For this review, use the dimensioned drawing (mm, ordinates from the lowest corner) and the shaded views. A direction names the side the tool comes from. Coordinates: 2 decimals unless noted, no trailing zeros. Order: outer loops, then holes, each group sorted by start corner. A loop starts at its lowest first (then second) coordinate and runs counter-clockwise, first axis right, second up. Notation, with made-up numbers: M -14,3.5 L 21,3.5 A24 cw 21,35.5 Z; hole C 88.25,-36 d7. An arc over 180 degrees is marked long. Answer as CSV lines item,"result". Start each with the question number.
Q1. Consider section D-D on x = 21. Write out the cut boundary in (y, z), and give its area (3 significant figures).
Q2. Wall thickness on L1, parallel to Y at x = 40, z = 33; L2, parallel to Y at x = 6.5, z = 26.5; L3, parallel to Y at x = 61, z = 32: over which ranges is each line inside the solid? List them lowest first. Write a range as [from, to].
Q3. Machinability: for the marked faces 5, 6 and 7, which of the approach directions +Z, -Z, +X, -X, +Y, -Y give a long, thin tool a straight path to every point of the face, cutting with its end or side? Answer none if there is none.
Q4. For P1, Ø4, axis at y = 65.5, z = 18.5, coming from the -X side; P2, Ø2, axis at y = 21.5, z = 28, coming from the -X side; P3, Ø21.5, axis at x = 51.5, z = 14.5, coming from the +Y side; P4, Ø4, axis at x = 42.5, y = 29.5, coming from the +Z side, all flat-tipped, find the tip position at first contact; note any pin that passes through.
Q5. Consider section A-A on x = 35. Write out the cut boundary in (y, z).
Q6. Consider section B-B on y = 26.5. Write out the cut boundary in (x, z).
Q7. Consider section C-C on z = 34.5. Write out the cut boundary in (x, y), and give its area (3 significant figures).
Q8. The part is to be moulded in two halves that separate along Y. For the marked faces 1, 2, 3 and 4, say which applies: +Y half, -Y half, draft (parallel to the pull), parting line (faces both ways), or undercut.
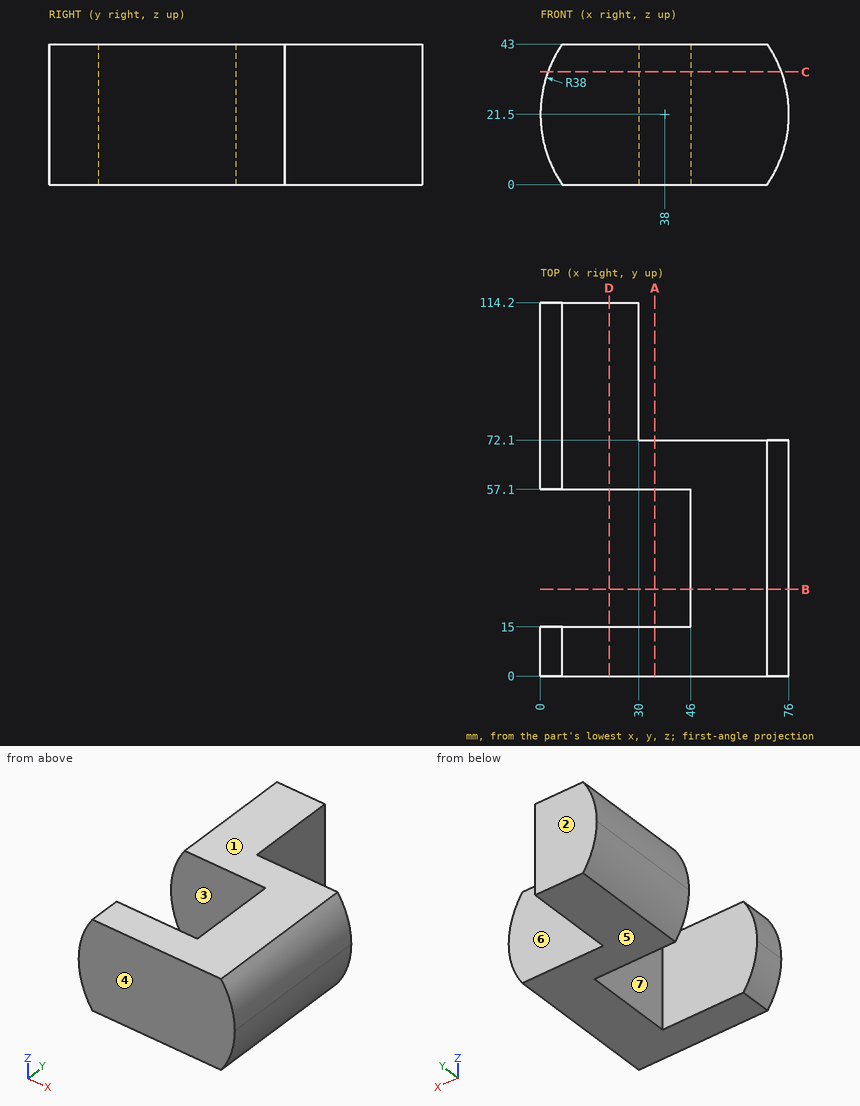
Evaluation:
1,outline,"M 0,0 L 15,0 L 15,43 L 0,43 Z; M 57.1,0 L 114.2,0 L 114.2,43 L 57.1,43 Z"
1,area,"3,100 mm²"
2,L1,"y = [0, 15], [57.1, 72.1]"
2,L2,"y = [0, 15], [57.1, 114.2]"
2,L3,"y = [0, 72.1]"
3,face 5,"-Z, +X, -X, +Y, -Y"
3,face 6,"+Z, -Z, +X, +Y"
3,face 7,"+Z, -Z, -X"
4,P1,"stops at x = 0.01"
4,P2,"stops at x = 46"
4,P3,"stops at y = 72.1"
4,P4,"passes through"
5,outline,"M 0,0 L 15,0 L 15,43 L 0,43 Z; M 57.1,0 L 72.1,0 L 72.1,43 L 57.1,43 Z"
6,outline,"M 46,0 L 69.33,0 A38 ccw 69.33,43 L 46,43 Z"
7,outline,"M 2.29,0 L 73.71,0 L 73.71,72.1 L 30,72.1 L 30,114.2 L 2.29,114.2 L 2.29,57.1 L 46,57.1 L 46,15 L 2.29,15 Z"
7,area,"4,480 mm²"
8,face 1,"draft"
8,face 2,"+Y half"
8,face 3,"undercut"
8,face 4,"-Y half"
